Part model, mm, in its own coordinate system. Round coordinates to 2 decimals unless told otherwise and drop trailing zeros. Answer as a JSON object with one key per item and string values.
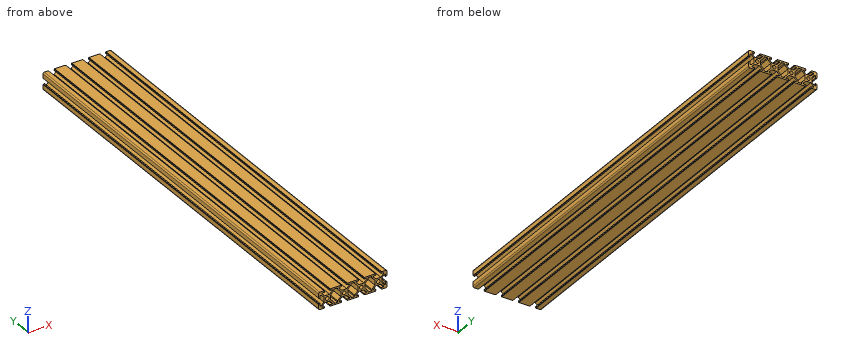
```python
from build123d import *

# Parameters (mm, degrees)
SKETCH_R          = 2.1
PAD_DEPTH         = 250
FILLET_R          = 1.5
SKETCH001_R       = 0.5
POCKET_DEPTH      = 250.001
POCKET_DEPTH_BACK = -250.001


with BuildPart() as part:
    # Sketch → Pad (new body, symmetric)
    with BuildSketch(Plane.XZ):
        Polygon((-10, 10), (-3.1, 10), (-3.1, 8.2), (-6, 8.2), (-6, 7.06066), (-2.83934, 3.9), (2.83934, 3.9), (6, 7.06066), (6, 8.2), (3.1, 8.2), (3.1, 10), (16.9, 10), (16.9, 8.2), (14, 8.2), (14, 7.06066), (17.16066, 3.9), (22.83934, 3.9), (26, 7.06066), (26, 8.2), (23.1, 8.2), (23.1, 10), (36.9, 10), (36.9, 8.2), (34, 8.2), (34, 7.06066), (37.16066, 3.9), (42.83934, 3.9), (46, 7.06066), (46, 8.2), (43.1, 8.2), (43.1, 10), (56.9, 10), (56.9, 8.2), (54, 8.2), (54, 7.06066), (57.16066, 3.9), (62.83934, 3.9), (66, 7.06066), (66, 8.2), (63.1, 8.2), (63.1, 10), (70, 10), (70, 3.1), (68.2, 3.1), (68.2, 6), (67.06066, 6), (63.9, 2.83934), (63.9, -2.83934), (67.06066, -6), (68.2, -6), (68.2, -3.1), (70, -3.1), (70, -10), (63.1, -10), (63.1, -8.2), (66, -8.2), (66, -7.06066), (62.83934, -3.9), (57.16066, -3.9), (54, -7.06066), (54, -8.2), (56.9, -8.2), (56.9, -10), (43.1, -10), (43.1, -8.2), (46, -8.2), (46, -7.06066), (42.83934, -3.9), (37.16066, -3.9), (34, -7.06066), (34, -8.2), (36.9, -8.2), (36.9, -10), (23.1, -10), (23.1, -8.2), (26, -8.2), (26, -7.06066), (22.83934, -3.9), (17.16066, -3.9), (14, -7.06066), (14, -8.2), (16.9, -8.2), (16.9, -10), (3.1, -10), (3.1, -8.2), (6, -8.2), (6, -7.06066), (2.83934, -3.9), (-2.83934, -3.9), (-6, -7.06066), (-6, -8.2), (-3.1, -8.2), (-3.1, -10), (-10, -10), (-10, -3.1), (-8.2, -3.1), (-8.2, -6), (-7.06066, -6), (-3.9, -2.83934), (-3.9, 2.83934), (-7.06066, 6), (-8.2, 6), (-8.2, 3.1), (-10, 3.1), align=None)
        Circle(SKETCH_R, mode=Mode.SUBTRACT)
        with Locations((20, 0)):
            Circle(SKETCH_R, mode=Mode.SUBTRACT)
        with Locations((40, 0)):
            Circle(SKETCH_R, mode=Mode.SUBTRACT)
        with Locations((59.9, 0)):
            Circle(SKETCH_R, mode=Mode.SUBTRACT)
        Polygon((7.8, -6.53934), (4.1, -2.83934), (4.1, 2.83934), (7.8, 6.53934), (7.8, 8.2), (12.2, 8.2), (12.2, 6.53934), (15.9, 2.83934), (15.9, -2.83934), (12.2, -6.53934), (12.2, -8.2), (7.8, -8.2), align=None, mode=Mode.SUBTRACT)
        Polygon((27.8, 8.2), (27.8, 6.53934), (24.1, 2.83934), (24.1, -2.83934), (27.8, -6.53934), (27.8, -8.2), (32.2, -8.2), (32.2, -6.53934), (35.9, -2.83934), (35.9, 2.83934), (32.2, 6.53934), (32.2, 8.2), align=None, mode=Mode.SUBTRACT)
        Polygon((47.8, 8.2), (47.8, 6.53934), (44.1, 2.83934), (44.1, -2.83934), (47.8, -6.53934), (47.8, -8.2), (52.2, -8.2), (52.2, -6.53934), (55.9, -2.83934), (55.9, 2.83934), (52.2, 6.53934), (52.2, 8.2), align=None, mode=Mode.SUBTRACT)
    extrude(amount=PAD_DEPTH, both=True)

    # Fillet
    fillet_edges = [part.edges().sort_by_distance(p)[0] for p in [
        (-10, 0, 10),
        (-10, 0, -10),
        (70, 0, -10),
        (70, 0, 10),
    ]]
    fillet(fillet_edges, radius=FILLET_R)

    # Sketch001 → Pocket (cut, two sides)
    with BuildSketch(Plane.XZ) as pocket_sk:
        with Locations((63.1, 10)):
            Circle(SKETCH001_R)
        with Locations((56.9, 10)):
            Circle(SKETCH001_R)
        with Locations((70, 3.1)):
            Circle(SKETCH001_R)
        with Locations((70, -3.1)):
            Circle(SKETCH001_R)
        with Locations((63.1, -10)):
            Circle(SKETCH001_R)
        with Locations((56.9, -10)):
            Circle(SKETCH001_R)
        with Locations((43.1, -10)):
            Circle(SKETCH001_R)
        with Locations((36.9, -10)):
            Circle(SKETCH001_R)
        with Locations((23.1, -10)):
            Circle(SKETCH001_R)
        with Locations((16.9, -10)):
            Circle(SKETCH001_R)
        with Locations((43.1, 10)):
            Circle(SKETCH001_R)
        with Locations((36.9, 10)):
            Circle(SKETCH001_R)
        with Locations((23.1, 10)):
            Circle(SKETCH001_R)
        with Locations((16.9, 10)):
            Circle(SKETCH001_R)
        with Locations((3.1, 10)):
            Circle(SKETCH001_R)
        with Locations((-3.1, 10)):
            Circle(SKETCH001_R)
        with Locations((-10, 3.1)):
            Circle(SKETCH001_R)
        with Locations((-10, -3.1)):
            Circle(SKETCH001_R)
        with Locations((-3.1, -10)):
            Circle(SKETCH001_R)
        with Locations((3.1, -10)):
            Circle(SKETCH001_R)
    extrude(amount=-POCKET_DEPTH, mode=Mode.SUBTRACT)
    extrude(pocket_sk.sketch, amount=-POCKET_DEPTH_BACK, mode=Mode.SUBTRACT)


with BuildPart() as part_1:
    # Body placement: moved
    add(part.part.moved(Location((-30, 0, 0))))


solid = part_1.part
```
Item 1: Cut at A-A (y = -142). State how many separate pieces and enclosed holes the cut face has, plus the area to 3 significant figures.
Taken from the geometry:
{"separate pieces": "1", "enclosed holes": "7", "area": "586 mm2"}
Item 2: Drop flat-ended pins along their axis: P1, Ø10, axis at x = 2, z = -3.5, coming from the +Y side; P2, Ø1.7, axis at x = 9, y = -88, coming from the +Z side; P3, Ø0.7, axis at y = 114.5, z = 9, coming from the +X side; P4, Ø1.5, axis at y = 89.5, z = 1, coming from the -X side. Give the stop position or say it passes through.
Taken from the geometry:
{"P1": "y = 250", "P2": "z = 3.9", "P3": "x = 39.99", "P4": "x = -33.9"}
Item 3: Probe L1, parallel to X at y = 177, z = 8.5; L2, parallel to X at y = 79, z = 2.5; L3, parallel to X at y = -138, z = -3.25. List the from-to ranges inside material, lowest first. Write a range as from..to.
Taken from the geometry:
{"L1": "-40..-33.1, -26.9..-13.1, -6.9..6.9, 13.1..26.9, 33.1..40", "L2": "-33.9..-25.9, -14.1..-5.9, 5.9..14.1, 25.9..33.9", "L3": "-39.52..-38.2, -34.31..-25.49, -14.51..-5.49, 5.49..14.51, 25.49..34.31, 38.2..39.52"}
